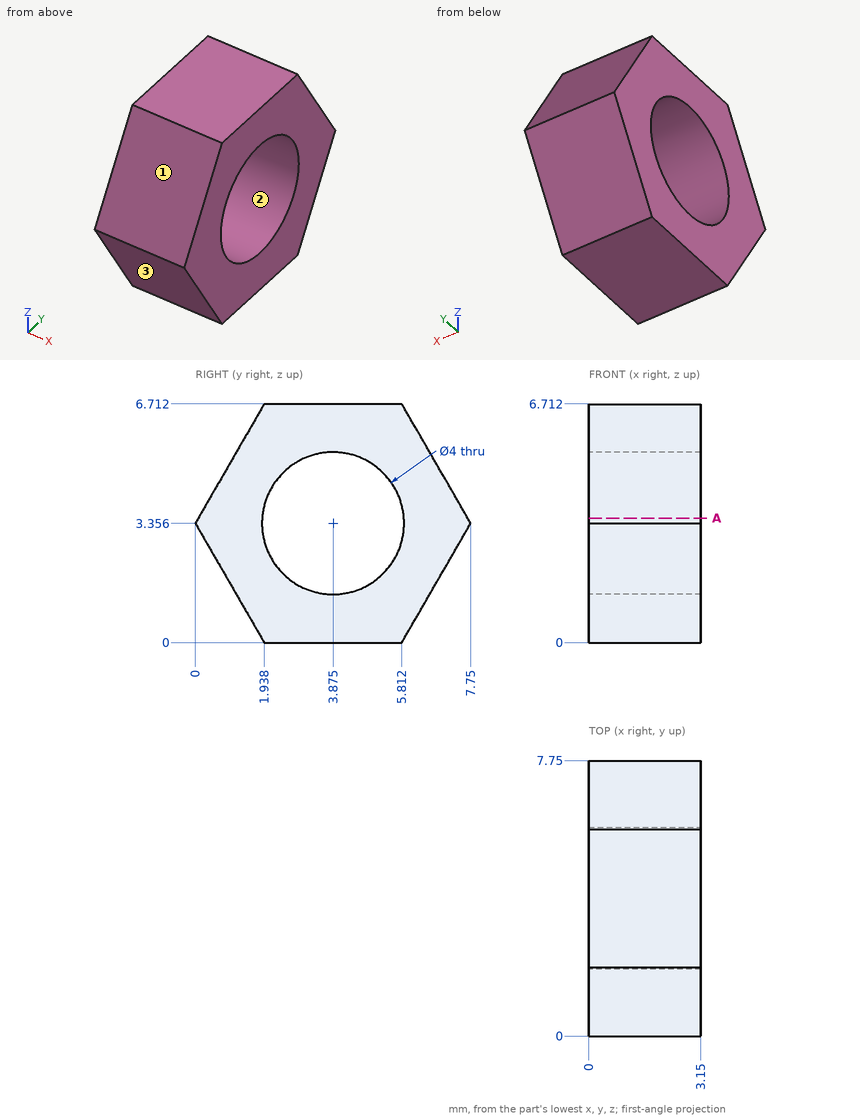
Input: dimensioned drawing with shaded views. Units: mm. Origin: part minimum x, y, z. Coordinates: 2 decimals unless noted, no trailing zeros. Loops run counter-clockwise (first coordinate to the right, second up) from the corner with the lowest first, then second, coordinate; pieces in that order, holes last. Notation, with made-up numbers: (30.25, 57.5) -> (49.25, 57.5) arc R30 ccw to (49.25, 92.5) -> close; hole circle Ø3 at (50, 79.5). An arc over 180 degrees is marked (long way). Use a Markdown table: item, result. Add a question column.
(1) Section query A-A, the plane z = 3.5. Return loops of the section in (x, y).
(2) Pin query (flat end, axial travel): pin 1 Ø1 at (x, z) = (0.5, 4.5) entering from -Y. Return the tip coordinate at first contact, or that it passes through.
(3) Mould query, pull axis Z, two halves, no side actions, for the marked faces 1, 2 and 3. Classes: pulls with the +Z half, pulls with the -Z half, needs draft (parallel to the pull), parting line crosses it, or undercut.
(4) Line query: line 1 along Y through (x, z) = (2.35, 3) (1 decimal); line 2 along Z through (x, y) = (0.6, 3) (1 decimal); line 3 along Y through (x, z) = (2.8, 4.25) (1 decimal). Output: solid intervals per line, ascending.
Answer:
| question | item | result |
|---|---|---|
| 1 | outline | (0, 0.08) -> (3.15, 0.08) -> (3.15, 1.88) -> (0, 1.88) -> close; (0, 5.87) -> (3.15, 5.87) -> (3.15, 7.67) -> (0, 7.67) -> close |
| 2 | pin 1 | stops at y = 0.37 |
| 3 | face 1 | pulls with the +Z half |
| 3 | face 2 | undercut |
| 3 | face 3 | pulls with the -Z half |
| 4 | line 1 | y = 0.2 to 1.9, 5.8 to 7.5 |
| 4 | line 2 | z = 0 to 1.6, 5.2 to 6.7 |
| 4 | line 3 | y = 0.5 to 2.1, 5.7 to 7.2 |
